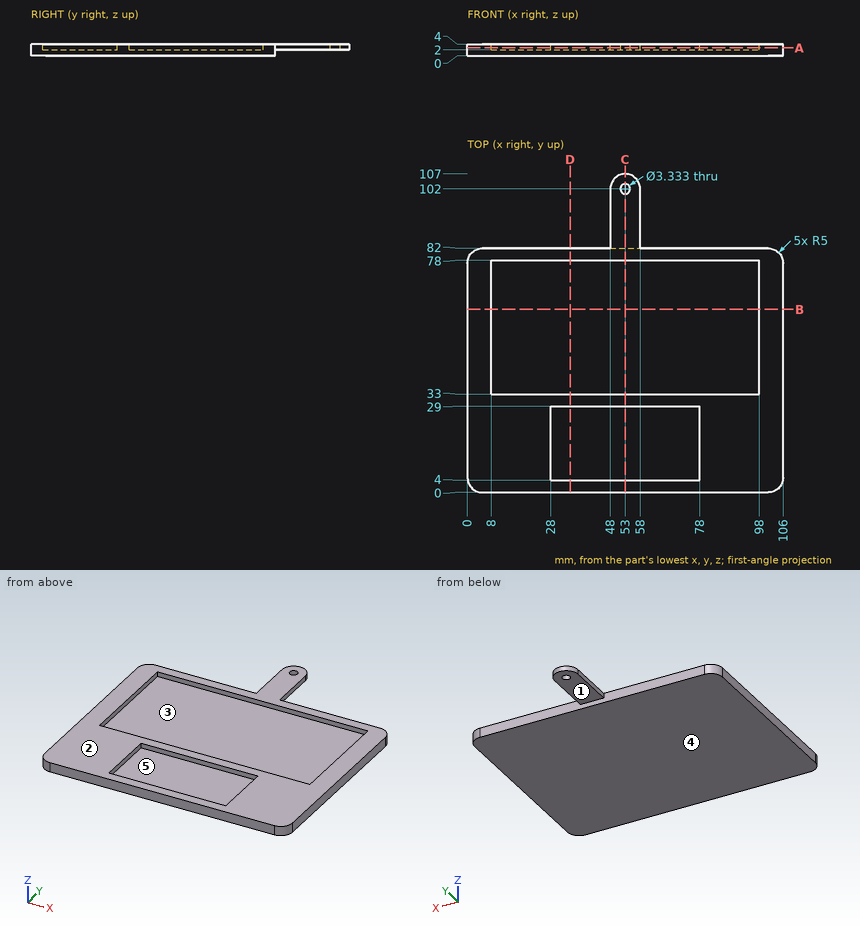
Print and shaded views of the part. All mm, measured from the part's lowest x, y and z. A direction names the side the tool comes from. Give positions to 0.01 mm unless a question says otherwise; leave off trailing zeros. Loops run counter-clockwise (first coordinate to the right, second up) from the corner with the lowest first, then second, coordinate; pieces in that order, holes last. Notation, with made-up numbers: (80.25, -26.5) -> (127.25, -26.5) arc R22 cw to (127.25, -10.5) -> close; hole circle Ø7 at (-16.5, -21.75). An arc over 180 degrees is marked (long way). Answer in a Markdown table with one row per item.
Item 1: Slice it at B-B on y = 61.5. Write the cut outline in (x, z).
Findings below:
| item | result |
|---|---|
| outline | (0, 0) -> (106, 0) -> (106, 4) -> (98, 4) -> (98, 2) -> (8, 2) -> (8, 4) -> (0, 4) -> close |
Item 2: Slice it at C-C on x = 53. Write the cut outline in (y, z).
Findings below:
| item | result |
|---|---|
| outline | (0, 0) -> (82, 0) -> (82, 2) -> (100.33, 2) -> (100.33, 4) -> (78, 4) -> (78, 2) -> (33, 2) -> (33, 4) -> (29, 4) -> (29, 2) -> (4, 2) -> (4, 4) -> (0, 4) -> close; (103.67, 2) -> (107, 2) -> (107, 4) -> (103.67, 4) -> close |
Item 3: Mould opens along X. For the marked faces 3, 4 and 5 say: pulls with the +X half, pulls with the -X half, needs draft (parallel to the pull), parting line crosses it, or undercut.
Findings below:
| item | result |
|---|---|
| face 3 | undercut |
| face 4 | needs draft |
| face 5 | undercut |
Item 4: Probe line 1 along Y through (x, z) = (53, 2.65); line 2 along X through (y, z) = (102, 2.65); line 3 along X through (y, z) = (56.5, 3.5). List the from-to ranges inside material, lowest first. Write a range as [from, to].
Findings below:
| item | result |
|---|---|
| line 1 | y = [0, 4], [29, 33], [78, 100.33], [103.67, 107] |
| line 2 | x = [48, 51.33], [54.67, 58] |
| line 3 | x = [0, 8], [98, 106] |
Item 5: Tool access for the marked faces 1 and 2: list every direction of +Z, -Z, +X, -X, +Y, -Y with a clear straight run to the whole face (end or side of a thin tool).
Findings below:
| item | result |
|---|---|
| face 1 | -Z, +X, -X, +Y |
| face 2 | +Z, +X, -X, +Y, -Y |
Item 6: Flat gauge pins, fed straight in: P1, Ø11, axis at x = 55, y = 95, coming from the -Z side; P2, Ø1, axis at y = 80, z = 1, coming from the +X side; P3, Ø1, axis at y = 93, z = 2.5, coming from the -X side. Where does each tip first touch, or does it go through?
Findings below:
| item | result |
|---|---|
| P1 | stops at z = 2 |
| P2 | stops at x = 105.33 |
| P3 | stops at x = 48 |
Item 7: Slice it at D-D on x = 34.5. Write the cut outline in (y, z).
Findings below:
| item | result |
|---|---|
| outline | (0, 0) -> (82, 0) -> (82, 4) -> (78, 4) -> (78, 2) -> (33, 2) -> (33, 4) -> (29, 4) -> (29, 2) -> (4, 2) -> (4, 4) -> (0, 4) -> close |
Item 8: Slice it at A-A on z = 2.7. Write the cut outline in (x, y).
Findings below:
| item | result |
|---|---|
| outline | (0, 5) arc R5 ccw to (5, 0) -> (101, 0) arc R5 ccw to (106, 5) -> (106, 77) arc R5 ccw to (101, 82) -> (58, 82) -> (58, 102) arc R5 ccw to (48, 102) -> (48, 82) -> (5, 82) arc R5 ccw to (0, 77) -> close; hole (8, 33) -> (98, 33) -> (98, 78) -> (8, 78) -> close; hole (28, 4) -> (78, 4) -> (78, 29) -> (28, 29) -> close; hole circle Ø3.33 at (53, 102) |
